Design review of the part shown in the three views and the two pictorial views. Dimensions are in mm from the part's minimum x, y and z. Round coordinates to 2 decimals unless told otherwise and drop trailing zeros. Order: outer loops, then holes, each group sorted by start corner. A loop starts at its lowest first (then second) coordinate and runs counter-clockwise, first axis right, second up.
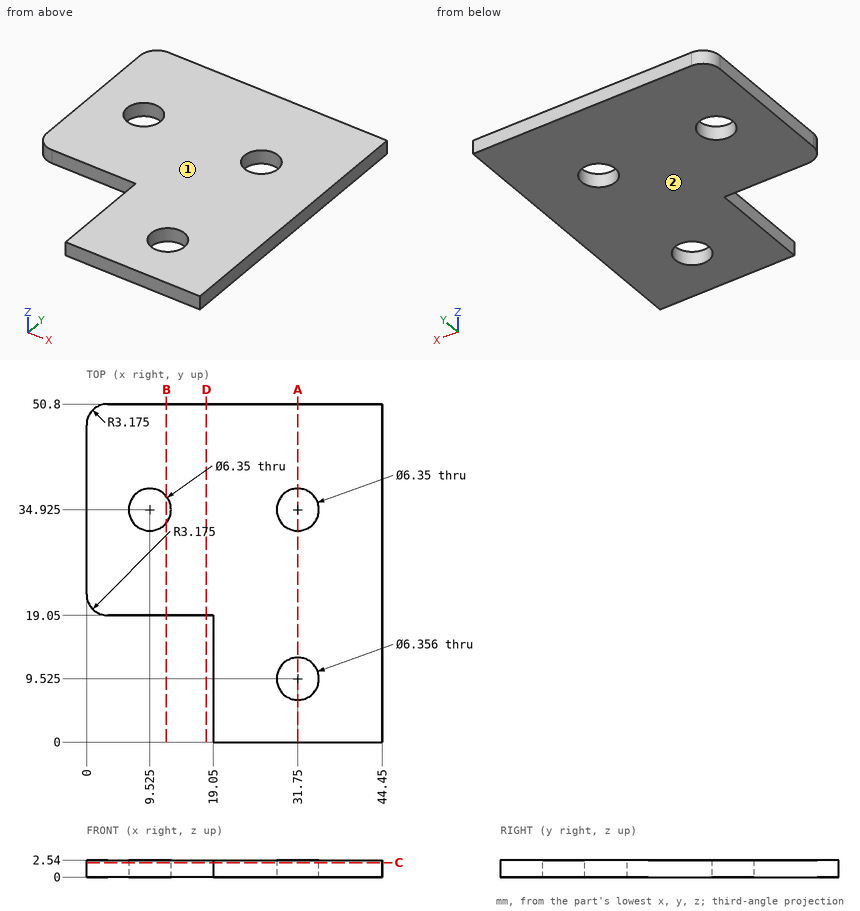
(1) Clearance check with a flat-ended pin moving along its axis: P1, Ø7.5, axis at x = 9.525, y = 34.925, coming from the +Z side. State where the tip first meets the part, or that it passes through.
(2) Draft analysis for pull direction Z (two halves, no side actions). For the marked faces 1 and 2, state which applies: pulls with the +Z half, pulls with the -Z half, needs draft (parallel to the pull), parting line crosses it, or undercut.
(3) Add section D-D on x = 18. Give the boundary of the cut face in (y, z).
(4) Add section B-B on x = 12. Give the boundary of the cut face in (y, z), plus the area to 3 significant figures.
(5) Add section A-A on x = 31.75. Give the boundary of the cut face in (y, z).
(6) Wall thickness on L1, parallel to Y at x = 31.75, z = 1.7; L2, parallel to Y at x = 29.5, z = 0.45; L3, parallel to X at y = 17.5, z = 0.55: over which ranges is each line inside the solid? List them lowest first.
(7) Add section C-C on z = 2.15. Give the boundary of the cut face in (x, y) (3 decimals).
Here are the results:
1. P1: stops at z = 2.54
2. face 1: pulls with the +Z half
2. face 2: pulls with the -Z half
3. outline: (19.05, 0) - (50.8, 0) - (50.8, 2.54) - (19.05, 2.54) - close
4. outline: (19.05, 0) - (32.94, 0) - (32.94, 2.54) - (19.05, 2.54) - close; (36.91, 0) - (50.8, 0) - (50.8, 2.54) - (36.91, 2.54) - close
4. area: 70.5 mm2
5. outline: (0, 0) - (6.35, 0) - (6.35, 2.54) - (0, 2.54) - close; (12.7, 0) - (31.75, 0) - (31.75, 2.54) - (12.7, 2.54) - close; (38.1, 0) - (50.8, 0) - (50.8, 2.54) - (38.1, 2.54) - close
6. L1: y = 0 to 6.35, 12.7 to 31.75, 38.1 to 50.8
6. L2: y = 0 to 7.28, 11.77 to 32.68, 37.17 to 50.8
6. L3: x = 19.05 to 44.45
7. outline: (0, 22.225) arc R3.175 ccw to (3.175, 19.05) - (19.05, 19.05) - (19.05, 0) - (44.45, 0) - (44.45, 50.8) - (3.175, 50.8) arc R3.175 ccw to (0, 47.625) - close; hole circle Ø6.35 at (9.525, 34.925); hole circle Ø6.356 at (31.75, 9.525); hole circle Ø6.35 at (31.75, 34.925)
